Check sheet for the drawn part. Datum: minimum x, y, z corner. Units: mm. Round coordinates to 2 decimals unless told otherwise and drop trailing zeros. Order: outer loops, then holes, each group sorted by start corner. A loop starts at its lowest first (then second) coordinate and runs counter-clockwise, first axis right, second up.
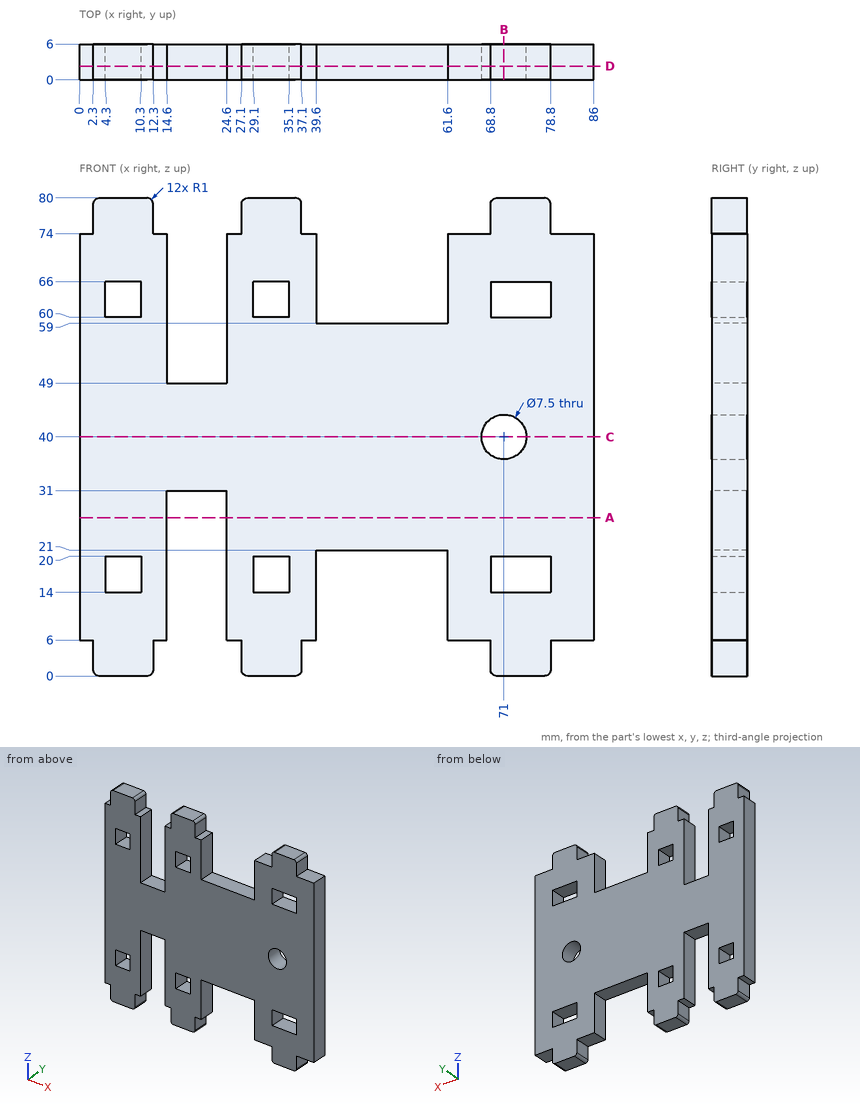
1) Sectioned sample at D-D on y = 2.3. Count the separate pieces of the cut face and the enclosed holes in it, and give its area (3 significant figures).
2) Gauge pin test, flat ends, axial feed: pin 1 (6 mm diameter, centred on x = 20, z = 40, fed in from -Y); pin 2 (3 mm diameter, centred on x = 21.5, y = 4, fed in from +Z); pin 3 (3 mm diameter, centred on x = 66, y = 3, fed in from -Z); pin 4 (2.5 mm diameter, centred on x = 1, y = 2, fed in from +Z). Record the tip position at first contact, or that the pin passes through.
3) Sectioned sample at C-C on z = 40. Record the cut outline in (x, y).
4) Scan lines: line 1 (Z direction, x = 7, y = 1.9); line 2 (X direction, y = 3.75, z = 76); line 3 (Z direction, x = 71, y = 1.45). Record each from-to range of solid material in increasing order.
5) Sectioned sample at A-A on z = 26.5. Record the cut outline in (x, y).
6) Sectioned sample at B-B on x = 71. Record the cut outline in (y, z).
Values found:
1. separate pieces: 1
1. enclosed holes: 7
1. area: 4,740 mm2
2. pin 1: stops at y = 0
2. pin 2: stops at z = 49
2. pin 3: stops at z = 6
2. pin 4: stops at z = 74
3. outline: (0, 0) - (67.25, 0) - (67.25, 6) - (0, 6) - close; (74.75, 0) - (86, 0) - (86, 6) - (74.75, 6) - close
4. line 1: z = 0 to 14, 20 to 60, 66 to 80
4. line 2: x = 2.3 to 12.3, 27.1 to 37.1, 68.8 to 78.8
4. line 3: z = 0 to 14, 20 to 36.25, 43.75 to 60, 66 to 80
5. outline: (0, 0) - (14.6, 0) - (14.6, 6) - (0, 6) - close; (24.6, 0) - (86, 0) - (86, 6) - (24.6, 6) - close
6. outline: (0, 0) - (6, 0) - (6, 14) - (0, 14) - close; (0, 20) - (6, 20) - (6, 36.25) - (0, 36.25) - close; (0, 43.75) - (6, 43.75) - (6, 60) - (0, 60) - close; (0, 66) - (6, 66) - (6, 80) - (0, 80) - close
